CAD build for the part. Positions are in the model's coordinates, mm. Face numbers are marked on the shaded views. A direction names the side the tool comes from. Give positions to 0.01 mm unless a question says otherwise; leave off trailing zeros. Write each loop counter-clockwise with the first axis right and the second up, starting at its lowest first coordinate (ties: lowest second). Pieces come first, ordered by that corner, then holes. Notation, with made-up numbers: M -35.5,2 L 22.5,2 A12 cw 22.5,15 Z; hole C -40,4 d10. An arc over 180 degrees is marked long. One line per question, with ' | ' between items. Start each with the question number.
1. Cut at C-C, the plane y = 13.56. Write the cut outline in (x, z), then the cut area to 3 significant figures.
2. Wall check: L1, parallel to Z at x = -17.5, y = -6; L2, parallel to Y at x = -15, z = 2; L3, parallel to X at y = 0, z = 19.55. Give the ranges that are in metal, low to high.
3. Flat gauge pins, fed straight in: pin 1 (9 mm diameter, centred on x = -4, z = 10.5, fed in from +Y); pin 2 (4.5 mm diameter, centred on y = 11.5, z = 13.5, fed in from -X); pin 3 (7.5 mm diameter, centred on y = 18.5, z = 13, fed in from +X); pin 4 (5 mm diameter, centred on x = 0, y = 0, fed in from +Z). Where does each tip first touch, or does it go through?
4. Pull direction Z, two halves, no side cores. Call the marked faces 1, 2 and 3: released by +Z, released by -Z, zero draft, split by the parting line, or undercut.
5. Which spindle directions (+Z, -Z, +X, -X, +Y, -Y) get a long thin tool onto all of the face, cutting with end or side? Do the marked faces 4, 5 and 6. Say none if no direction does.
6. Cut at A-A, the plane z = 2. Write the cut outline in (x, y), then the cut area to 3 significant figures.
7. Cut at D-D, the plane y = 0. Write the cut outline in (x, z), then the cut area to 3 significant figures.
8. Cut at B-B, the plane x = -17.94. Write the cut outline in (y, z), then the cut area to 3 significant figures.
```python
from build123d import *

# Parameters (mm, degrees)
SKETCH4_R           = 3
BOSS_EXTRUDE1_DEPTH = 20
SKETCH5_W           = 18
SKETCH5_H           = 16
CUT_EXTRUDE3_DEPTH  = 36.94
SKETCH6_W           = 18
SKETCH6_H           = 14.56
CUT_EXTRUDE4_DEPTH  = 17


with BuildPart() as part:
    # Sketch4 → Boss-Extrude1 (new body)
    with BuildSketch(Plane.XY):
        Polygon((-8.94, 9), (-8.94, 23.56), (-26.94, 23.56), (-26.94, -9), (9, -9), (9, 9), align=None)
        Circle(SKETCH4_R, mode=Mode.SUBTRACT)
        with Locations((-17.94, 13.56)):
            Circle(SKETCH4_R, mode=Mode.SUBTRACT)
    extrude(amount=BOSS_EXTRUDE1_DEPTH)

    # Sketch5 → Cut-Extrude3 (cut, through all)
    with BuildSketch(Plane(origin=(9, 0, 0), x_dir=(0, 0, -1), z_dir=(1, 0, 0))):
        with Locations((-10, 0)):
            Rectangle(SKETCH5_W, SKETCH5_H)
    extrude(amount=-CUT_EXTRUDE3_DEPTH, mode=Mode.SUBTRACT)

    # Sketch6 → Cut-Extrude4 (cut)
    with BuildSketch(Plane.ZY.offset(26.94)):
        with Locations((10, 15.28)):
            Rectangle(SKETCH6_W, SKETCH6_H)
    extrude(amount=-CUT_EXTRUDE4_DEPTH, mode=Mode.SUBTRACT)


solid = part.part
```
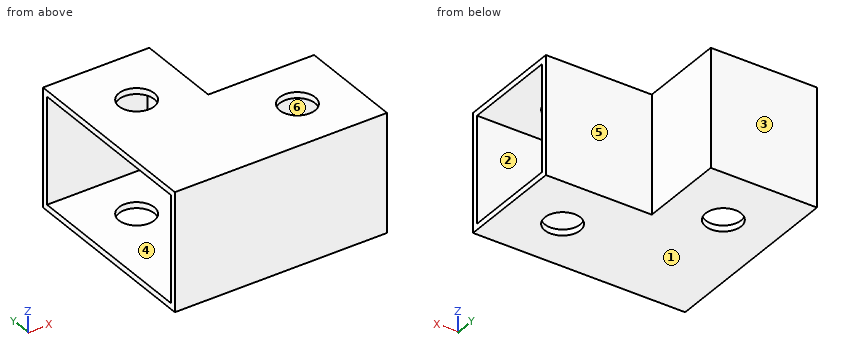
Here are the results:
1) outline: M -26.94,0 L -20.94,0 L -20.94,1 L -26.94,1 Z; M -26.94,19 L -20.94,19 L -20.94,20 L -26.94,20 Z; M -14.94,0 L -8.94,0 L -8.94,20 L -14.94,20 L -14.94,19 L -9.94,19 L -9.94,1 L -14.94,1 Z | area: 42.0 mm^2
2) L1: 0 to 1, 19 to 20 | L2: -9 to -8, 22.56 to 23.56 | L3: -26.94 to -3, 3 to 9
3) pin 1: y = 9 | pin 2: x = -9.94 | pin 3: x = -8.94 | pin 4: through
4) face 1: released by -Z | face 2: undercut | face 3: zero draft
5) face 4: -X | face 5: +Z, -Z, +X, +Y | face 6: +X, -X
6) outline: M -26.94,-9 L 9,-9 L 9,-8 L -26.94,-8 Z; M -26.94,22.56 L -9.94,22.56 L -9.94,8 L 9,8 L 9,9 L -8.94,9 L -8.94,23.56 L -26.94,23.56 Z | area: 86.4 mm^2
7) outline: M -26.94,0 L -3,0 L -3,1 L -26.94,1 Z; M -26.94,19 L -3,19 L -3,20 L -26.94,20 Z; M 3,0 L 9,0 L 9,1 L 3,1 Z; M 3,19 L 9,19 L 9,20 L 3,20 Z | area: 59.9 mm^2
8) outline: M -9,0 L 10.56,0 L 10.56,1 L -8,1 L -8,19 L 10.56,19 L 10.56,20 L -9,20 Z; M 16.56,0 L 23.56,0 L 23.56,20 L 16.56,20 L 16.56,19 L 22.56,19 L 22.56,1 L 16.56,1 Z | area: 89.1 mm^2
